Read the model definition and answer for the solid it produces. Units are mm, in the model's axes. A direction names the side the tool comes from. Give positions to 0.01 mm unless a question says otherwise; leave off trailing zeros. Write each loop counter-clockwise with the first axis right and the second up, starting at its lowest first coordinate (ties: lowest second). Pieces come first, ordered by that corner, then holes. Notation, with made-up numbers: M 81.25,70.5 L 115.25,70.5 A34 cw 115.25,105.5 Z; hole C 34,41.25 d7. An arc over 180 degrees is marked long. Use a Markdown table: item, result. Add a question column.
Item 1: A cutting plane is placed at C-C on y = 4.25. Determine the outline of the cut face in (x, z), then the cut area to 3 significant figures.
Item 2: Consider probe 1 along Z at (x, y) = (-5, -5); probe 2 along Y at (x, z) = (4, 16.5); probe 3 along X at (y, z) = (4, 13.5). Determine where each line is inside the solid, lowest interval first. Write a range as [from, to].
Item 3: The mould has two halves that part along X. Classify faces 3 (the cylindrical face through (-15.215, -0.106, 14.79)), 4 (the flat face through (0, -10, 15)), 5 (the cylindrical face through (-18.998, 9.049, 14.79)): pulls with the +X half, pulls with the -X half, needs draft (parallel to the pull), parting line crosses it, or undercut.
Item 4: A cutting plane is placed at A-A on x = 5.5. Determine the outline of the cut face in (y, z).
Item 5: For faces 1 (the flat face through (20, -5, 15)), 2 (the flat face through (5, -3, 15)), determine the directions among +Z, -Z, +X, -X, +Y, -Y from which every point of the face is accessible in a straight line to the end or side of a thin tool.
Item 6: A cutting plane is placed at D-D on z = 15.5. Count the separate pieces of the cut face and the enclosed holes in it, then the cut area to 3 significant figures.
Item 7: A cutting plane is placed at B-B on x = 15. Determine the outline of the cut face in (y, z).
from build123d import *

# Parameters (mm, degrees)
F1_DEPTH = 30
F2_R     = 3.05
F3_DEPTH = 30


with BuildPart() as f1:
    # F0 (on Top) → F1 (new body)
    with BuildSketch(Plane.XY):
        with BuildLine():
            Line((-20, 6.6666666667), (-20, -6.6666666667))
            ThreePointArc((-20, -6.6666666667), (-19.0236892706, -9.0236892706), (-16.6666666667, -10))
            Line((-16.6666666667, -10), (16.6666666667, -10))
            ThreePointArc((16.6666666667, -10), (19.0236892706, -9.0236892706), (20, -6.6666666667))
            Line((20, -6.6666666667), (20, -3))
            Line((20, -3), (-9.7565921577, -3))
            Line((-9.7565921577, -3), (-9.7565921577, -2.9923427896))
            ThreePointArc((-9.7565921577, -2.9923427896), (-15.2166666667, 0), (-9.7565921577, 2.9923427896))
            Line((-9.7565921577, 2.9923427896), (-9.7565921577, 3))
            Line((-9.7565921577, 3), (20, 3))
            Line((20, 3), (20, 6.6666666667))
            ThreePointArc((20, 6.6666666667), (19.0236892706, 9.0236892706), (16.6666666667, 10))
            Line((16.6666666667, 10), (-16.6666666667, 10))
            ThreePointArc((-16.6666666667, 10), (-19.0236892706, 9.0236892706), (-20, 6.6666666667))
        make_face()
    extrude(amount=F1_DEPTH)

    # F2 (on face) → F3 (cut)
    with BuildSketch(Plane.XZ.offset(10)):
        with Locations((-5, 15)):
            Circle(F2_R)
        with BuildLine():
            Line((16.6666666667, 12.5055617422), (16.6666666667, 17.4944382578))
            ThreePointArc((16.6666666667, 17.4944382578), (12, 15), (16.6666666667, 12.5055617422))
        make_face()
        with BuildLine():
            ThreePointArc((16.6666666667, 12.5055617422), (17.6457513111, 13.5857864376), (18, 15))
            ThreePointArc((18, 15), (17.6457513111, 16.4142135624), (16.6666666667, 17.4944382578))
            Line((16.6666666667, 17.4944382578), (16.6666666667, 12.5055617422))
        make_face()
    extrude(amount=-F3_DEPTH, mode=Mode.SUBTRACT)


solid = f1.part
Filled in:
| question | item | result |
|---|---|---|
| 1 | outline | M -20,0 L 20,0 L 20,30 L -20,30 Z; hole C -5,15 d6.1; hole C 15,15 d6 |
| 1 | area | 1,140 mm² |
| 2 | probe 1 | [0, 11.95], [18.05, 30] |
| 2 | probe 2 | [-10, -3], [3, 10] |
| 2 | probe 3 | [-20, -7.66], [-2.34, 12.4], [17.6, 20] |
| 3 | face 3 | undercut |
| 3 | face 4 | needs draft |
| 3 | face 5 | pulls with the -X half |
| 4 | outline | M -10,0 L -3,0 L -3,30 L -10,30 Z; M 3,0 L 10,0 L 10,30 L 3,30 Z |
| 5 | face 1 | +Z, -Z, +X, +Y, -Y |
| 5 | face 2 | +Z, -Z, +X |
| 6 | separate pieces | 5 |
| 6 | enclosed holes | 0 |
| 6 | area | 412 mm² |
| 7 | outline | M -10,0 L -3,0 L -3,12 L -10,12 Z; M -10,18 L -3,18 L -3,30 L -10,30 Z; M 3,0 L 10,0 L 10,12 L 3,12 Z; M 3,18 L 10,18 L 10,30 L 3,30 Z |
